from build123d import *

# Parameters (mm, degrees)
F1_DEPTH = 25.4
F2_DEPTH = 12.7
F4_DEPTH = 101.6


with BuildPart() as f1:
    # F0 (on Front) → F1 (new body, symmetric)
    with BuildSketch(Plane.XZ):
        with BuildLine():
            Line((44.9795118183, 19.6340414269), (-74.7879317753, -2.009495511))
            Line((-74.7879317753, -2.009495511), (-42.1710492869, -16.8047615714))
            ThreePointArc((-42.1710492869, -16.8047615714), (-28.2356794376, -5.2842052737), (-15.8599317753, -18.4659585731))
            Line((-15.8599317753, -18.4659585731), (23.9040682247, -18.4659585731))
            ThreePointArc((23.9040682247, -18.4659585731), (37.1120682247, -5.2579585731), (50.3200682247, -18.4659585731))
            Line((50.3200682247, -18.4659585731), (53.351612715, -18.4659585731))
            Line((53.351612715, -18.4659585731), (75.2120682247, 0))
            Line((75.2120682247, 0), (44.9795118183, 19.6340414269))
        make_face()
        with BuildLine():
            ThreePointArc((50.3200682247, -18.4659585731), (37.1120682247, -5.2579585731), (23.9040682247, -18.4659585731))
            Line((23.9040682247, -18.4659585731), (28.6366716027, -18.4659585731))
            Line((28.6366716027, -18.4659585731), (33.2120682247, -18.4659585731))
            ThreePointArc((33.2120682247, -18.4659585731), (37.1120682247, -14.5659585731), (41.0120682247, -18.4659585731))
            Line((41.0120682247, -18.4659585731), (45.5874648466, -18.4659585731))
            Line((45.5874648466, -18.4659585731), (50.3200682247, -18.4659585731))
        make_face()
        with BuildLine():
            ThreePointArc((-15.8599317753, -18.4659585731), (-28.2356794376, -5.2842052737), (-42.1710492869, -16.8047615714))
            Line((-42.1710492869, -16.8047615714), (-38.5088598291, -18.4659585731))
            Line((-38.5088598291, -18.4659585731), (-32.9679317753, -18.4659585731))
            ThreePointArc((-32.9679317753, -18.4659585731), (-29.0679317753, -14.5659585731), (-25.1679317753, -18.4659585731))
            Line((-25.1679317753, -18.4659585731), (-19.6270037216, -18.4659585731))
            Line((-19.6270037216, -18.4659585731), (-15.8599317753, -18.4659585731))
        make_face()
        with BuildLine():
            Line((-32.9679317753, -18.4659585731), (-38.5088598291, -18.4659585731))
            ThreePointArc((-38.5088598291, -18.4659585731), (-29.0679317753, -27.9068866268), (-19.6270037216, -18.4659585731))
            Line((-19.6270037216, -18.4659585731), (-25.1679317753, -18.4659585731))
            ThreePointArc((-25.1679317753, -18.4659585731), (-29.0679317753, -22.3659585731), (-32.9679317753, -18.4659585731))
        make_face()
        with BuildLine():
            Line((33.2120682247, -18.4659585731), (28.6366716027, -18.4659585731))
            ThreePointArc((28.6366716027, -18.4659585731), (37.1120682247, -26.941355195), (45.5874648466, -18.4659585731))
            Line((45.5874648466, -18.4659585731), (41.0120682247, -18.4659585731))
            ThreePointArc((41.0120682247, -18.4659585731), (37.1120682247, -22.3659585731), (33.2120682247, -18.4659585731))
        make_face()
    extrude(amount=F1_DEPTH, both=True)

    # F0 (on Front) → F2 (join, symmetric)
    with BuildSketch(Plane.XZ):
        with BuildLine():
            ThreePointArc((-15.8599317753, -18.4659585731), (-28.2356794376, -5.2842052737), (-42.1710492869, -16.8047615714))
            Line((-42.1710492869, -16.8047615714), (-38.5088598291, -18.4659585731))
            Line((-38.5088598291, -18.4659585731), (-32.9679317753, -18.4659585731))
            ThreePointArc((-32.9679317753, -18.4659585731), (-29.0679317753, -14.5659585731), (-25.1679317753, -18.4659585731))
            Line((-25.1679317753, -18.4659585731), (-19.6270037216, -18.4659585731))
            Line((-19.6270037216, -18.4659585731), (-15.8599317753, -18.4659585731))
        make_face()
        with BuildLine():
            ThreePointArc((50.3200682247, -18.4659585731), (37.1120682247, -5.2579585731), (23.9040682247, -18.4659585731))
            Line((23.9040682247, -18.4659585731), (28.6366716027, -18.4659585731))
            Line((28.6366716027, -18.4659585731), (33.2120682247, -18.4659585731))
            ThreePointArc((33.2120682247, -18.4659585731), (37.1120682247, -14.5659585731), (41.0120682247, -18.4659585731))
            Line((41.0120682247, -18.4659585731), (45.5874648466, -18.4659585731))
            Line((45.5874648466, -18.4659585731), (50.3200682247, -18.4659585731))
        make_face()
    extrude(amount=F2_DEPTH, both=True)

    # F3 (on Top) → F4 (cut, symmetric)
    with BuildSketch(Plane.XY):
        Polygon((0, -25.4), (-74.7879317753, 0), (0, 25.4), (0, 56.2246665359), (-99.1614311934, 56.2246665359), (-99.1614311934, -55.5053986609), (0, -55.5053986609), align=None)
    extrude(amount=F4_DEPTH, both=True, mode=Mode.SUBTRACT)


solid = f1.part
Input: part model. Units: mm. Frame: model coordinates. A direction names the side the tool comes from. Coordinates: 2 decimals unless noted, no trailing zeros. Loops run counter-clockwise (first coordinate to the right, second up) from the corner with the lowest first, then second, coordinate; pieces in that order, holes last. Notation, with made-up numbers: (-19, 35.5) - (-12, 35.5) arc R11 cw to (-12, 51.5) - close; hole circle Ø2 at (87.25, -26.75). An arc over 180 degrees is marked (long way). Answer in a Markdown table with one row per item. Add a question column.
Item 1: Line query: line 1 along X through (y, z) = (-3, -15.5); line 2 along Z through (x, y) = (40, 5.5); line 3 along X through (y, z) = (-1.5, -24). Output: solid intervals per line, ascending. Write a range as [from, to].
Item 2: Section query A-A on y = 9. Return the cut outline in (x, z), then the cut area to 3 significant figures.
Item 3: Contact query for flat-ended pins moving along their axis: P1, Ø5, axis at y = -7.5, z = 10.5, coming from the +X side; P2, Ø5, axis at x = 44, y = 4.5, coming from the +Z side; P3, Ø10, axis at x = -25.5, z = 6.5, coming from the -Y side. Output: stop coordinate, or through.
Item 4: Access query for faces 4 (the flat face through (4, 0, -18.466)), 5 (the flat face through (49, 0, -18.466)), 6 (the flat face through (-28.56, -15.7, -7.92)). Directions: +Z, -Z, +X, -X, +Y, -Y. A direction counts if a zero-diameter tool reaches every point of the face in a straight line with its end or side. Return the directions, or none.
Item 5: Mould query, pull axis X, two halves, no side actions, for faces 1 (the cylindrical face through (-29.276, -0.262, -27.905)), 2 (the flat face through (-0.76, -0.36, 11.37)), 3 (the flat face through (37, 25.4, -3)). Classes: released by +X, released by -X, zero draft, split by the parting line, or undercut.
Item 6: Section query B-B on z = 2. Return the cut outline in (x, y), then the cut area to 3 significant figures.
Item 7: Section query D-D on z = -8.5. Return the cut outline in (x, y).
Item 8: Section query C-C on x = -44.5. Return the cut outline in (y, z), then the cut area to 3 significant figures.
Recorded:
| question | item | result |
|---|---|---|
| 1 | line 1 | [-45.05, -31.6], [-26.54, 34.58], [39.64, 56.86] |
| 1 | line 2 | [-26.43, -21.09], [-15.84, 18.73] |
| 1 | line 3 | [-36.72, -21.42], [30.69, 43.53] |
| 2 | outline | (-48.29, -14.03) - (-38.51, -18.47) arc R9.44 ccw to (-19.63, -18.47) - (28.64, -18.47) arc R8.48 ccw to (45.59, -18.47) - (53.35, -18.47) - (75.21, 0) - (44.98, 19.63) - (-48.29, 2.78) - close; hole circle Ø7.8 at (-29.07, -18.47); hole circle Ø7.8 at (37.11, -18.47) |
| 2 | area | 3,560 mm^2 |
| 3 | P1 | x = 62.89 |
| 3 | P2 | z = 19.63 |
| 3 | P3 | y = -18.44 |
| 4 | face 4 | -Z, +Y, -Y |
| 4 | face 5 | -Z, +X, +Y, -Y |
| 4 | face 6 | +Z, -Z, -X, -Y |
| 5 | face 1 | undercut |
| 5 | face 2 | released by -X |
| 5 | face 3 | zero draft |
| 6 | outline | (-52.6, -7.54) - (0, -25.4) - (72.13, -25.4) - (72.13, 25.4) - (0, 25.4) - (-52.6, 7.54) - close |
| 6 | area | 5,400 mm^2 |
| 7 | outline | (-60.48, -4.86) - (0, -25.4) - (65.15, -25.4) - (65.15, 25.4) - (0, 25.4) - (-60.48, 4.86) - close |
| 8 | outline | (-10.29, -15.75) - (10.29, -15.75) - (10.29, 3.46) - (-10.29, 3.46) - close |
| 8 | area | 395 mm^2 |
